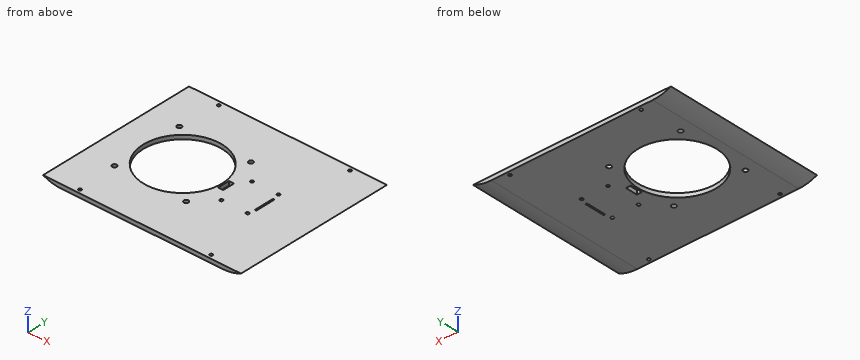
from build123d import *

# Parameters (mm, degrees)
SCHIZZO1_W                   = 160
SCHIZZO1_H                   = 160
SCHIZZO1_R                   = 1.5
ESTRUSIONE_ESTRUSIONE1_DEPTH = 4
SCHIZZO2_R                   = 1.5
SCHIZZO2_W                   = 1.5
SCHIZZO2_H                   = 20
TAGLIO_ESTRUSIONE1_DEPTH     = 36
SCHIZZO3_R                   = 39
SCHIZZO3_R_2                 = 2.25
SCHIZZO3_W                   = 5
SCHIZZO3_H                   = 12
TAGLIO_ESTRUSIONE2_DEPTH     = 7
SCHIZZO4_W                   = 4
SCHIZZO4_H                   = 160
ESTRUSIONE_ESTRUSIONE2_DEPTH = 18.13835714
SCHIZZO5_W                   = 4
SCHIZZO5_H                   = 160
ESTRUSIONE_ESTRUSIONE3_DEPTH = 18.13835714
TAGLIO_ESTRUSIONE3_DEPTH     = 229.13835714


with BuildPart() as part:
    # Schizzo1 → Estrusione-Estrusione1 (new body)
    with BuildSketch(Plane.XY):
        with Locations((-3.483874863, 13.01)):
            Rectangle(SCHIZZO1_W, SCHIZZO1_H)
        with Locations((-68.483874863, 89.01)):
            Circle(SCHIZZO1_R, mode=Mode.SUBTRACT)
        with Locations((61.516125137, 89.01)):
            Circle(SCHIZZO1_R, mode=Mode.SUBTRACT)
        with Locations((-68.483874863, -62.99)):
            Circle(SCHIZZO1_R, mode=Mode.SUBTRACT)
        with Locations((61.516125137, -62.99)):
            Circle(SCHIZZO1_R, mode=Mode.SUBTRACT)
    extrude(amount=ESTRUSIONE_ESTRUSIONE1_DEPTH)

    # Schizzo2 → Taglio-Estrusione1 (cut)
    with BuildSketch(Plane(origin=(0, 0, 0), x_dir=(-1, 0, 0), z_dir=(0, 0, -1))):
        with Locations((-44.071905048, 29.8436475)):
            Circle(SCHIZZO2_R)
        with Locations((-44.071905048, -3.8236475)):
            Circle(SCHIZZO2_R)
        with Locations((-18.082922837, -3.8236475)):
            Circle(SCHIZZO2_R)
        with Locations((-18.082922837, 29.8436475)):
            Circle(SCHIZZO2_R)
        with Locations((-45.766125137, 13.01)):
            Rectangle(SCHIZZO2_W, SCHIZZO2_H)
    extrude(amount=-TAGLIO_ESTRUSIONE1_DEPTH, mode=Mode.SUBTRACT)

    # Schizzo3 → Taglio-Estrusione2 (cut)
    with BuildSketch(Plane(origin=(0, 0, 0), x_dir=(-1, 0, 0), z_dir=(0, 0, -1))):
        with Locations((35.483874863, 13.01)):
            Circle(SCHIZZO3_R)
        with Locations((70.98387486, 48.509999997)):
            Circle(SCHIZZO3_R_2)
        with Locations(Location((70.98387486, -22.489999997, 0), (0, 0, 180))):
            Circle(SCHIZZO3_R_2)
        with Locations(Location((-0.016125134, 48.509999997, 0), (0, 0, 180))):
            Circle(SCHIZZO3_R_2)
        with Locations((-0.016125134, -22.489999997)):
            Circle(SCHIZZO3_R_2)
        with Locations((-7.516125137, 13.01)):
            Rectangle(SCHIZZO3_W, SCHIZZO3_H)
    extrude(amount=-TAGLIO_ESTRUSIONE2_DEPTH, mode=Mode.SUBTRACT)

    # Schizzo4 → Estrusione-Estrusione2 (add)
    with BuildSketch(Plane.ZY.offset(83.483874863)):
        with Locations((2, 13.01)):
            Rectangle(SCHIZZO4_W, SCHIZZO4_H)
    extrude(amount=ESTRUSIONE_ESTRUSIONE2_DEPTH)

    # Schizzo5 → Estrusione-Estrusione3 (add)
    with BuildSketch(Plane(origin=(76.516125137, 0, 0), x_dir=(0, 0, -1), z_dir=(1, 0, 0))):
        with Locations((-2, 13.01)):
            Rectangle(SCHIZZO5_W, SCHIZZO5_H)
    extrude(amount=ESTRUSIONE_ESTRUSIONE3_DEPTH)

    # Schizzo6 → Taglio-Estrusione3 (cut)
    with BuildSketch(Plane(origin=(0, 93.01, 0), x_dir=(1, 0, 0), z_dir=(0, 1, 0))):
        with BuildLine():
            Line((-101.622232003, -4), (-101.622232003, 0))
            Line((-101.622232003, 0), (-83.483874863, 0))
            ThreePointArc((-83.483874863, 0), (-92.77096267, -1.011871109), (-101.622232003, -4))
        make_face()
        with BuildLine():
            Line((76.516125137, 0), (94.654482277, 0))
            Line((94.654482277, 0), (94.654482277, -4))
            ThreePointArc((94.654482277, -4), (85.803212944, -1.011871109), (76.516125137, 0))
        make_face()
    extrude(amount=-TAGLIO_ESTRUSIONE3_DEPTH, mode=Mode.SUBTRACT)


solid = part.part
Verification items for the finished model (mm, model axes). Coordinates: 2 decimals unless noted, no trailing zeros. Order: outer loops, then holes, each group sorted by start corner. A loop starts at its lowest first (then second) coordinate and runs counter-clockwise, first axis right, second up. Notation, with made-up numbers: (-1, 78.25) -> (10, 78.25) arc R18 cw to (10, 88.25) -> close; hole circle Ø1 at (47.25, -0.5). An arc over 180 degrees is marked (long way). Put each result on its own line as item: value. Start each with the question number.
1. Cross-section at B-B, the plane z = 3.2. Count the separate pieces of the cut face and the enclosed holes in it, then the cut area to 3 significant figures.
2. Material ranges on L1, parallel to X at y = 3.5, z = 3.15; L2, parallel to Y at x = 6, z = 2.45; L3, parallel to Y at x = -2, z = 1.4, recorded low to high. Write a range as [from, to].
3. Cross-section at D-D, the plane y = -43. Record the boundary of the cut face in (x, z) (3 decimals).
4. Go/stop test with a flat-tipped pin: pin 1 Ø7 at (x, y) = (0.02, 48.51) entering from +Z. Record where the tip stops, or that it passes through.
5. Cross-section at C-C, the plane y = -13. Record the boundary of the cut face in (x, z) (3 decimals).
6. Cross-section at A-A, the plane y = 13.01. Record the boundary of the cut face in (x, z) (3 decimals), then the cut area to 3 significant figures.
Computed:
1. separate pieces: 1
1. enclosed holes: 15
1. area: 25,800 mm2
2. L1: [-99.66, -73.31], [2.34, 45.02], [46.52, 92.7]
2. L2: [-66.99, 7.01], [19.01, 93.01]
2. L3: [-66.99, -23.49], [-21.49, -6.99], [33.01, 47.51], [49.51, 93.01]
3. outline: (-101.622, 4) arc R43.125 ccw to (-83.484, 0) -> (76.516, 0) arc R43.125 ccw to (94.654, 4) -> close
4. pin 1: z = 4
5. outline: (-101.622, 4) arc R43.125 ccw to (-83.484, 0) -> (-64.544, 0) -> (-64.544, 4) -> close; (-6.424, 0) -> (76.516, 0) arc R43.125 ccw to (94.654, 4) -> (-6.424, 4) -> close
6. outline: (-101.622, 4) arc R43.125 ccw to (-83.484, 0) -> (-74.484, 0) -> (-74.484, 4) -> close; (3.516, 0) -> (5.016, 0) -> (5.016, 4) -> (3.516, 4) -> close; (10.016, 0) -> (45.016, 0) -> (45.016, 4) -> (10.016, 4) -> close; (46.516, 0) -> (76.516, 0) arc R43.125 ccw to (94.654, 4) -> (46.516, 4) -> close
6. area: 400 mm2
